from build123d import *

# Parameters (mm, degrees)
ESQUISSE1_W             = 48
ESQUISSE1_H             = 38
BOSS_EXTRU_1_DEPTH      = 8
ESQUISSE4_W             = 14
ESQUISSE4_H             = 15
ENL_V_MAT_EXTRU_2_DEPTH = 8
D_GAGEMENT_M41_D        = 4.3
D_GAGEMENT_M41_DEPTH    = 10
D_GAGEMENT_M41_TIP      = 1.291850331


with BuildPart() as part:
    # Esquisse1 → Boss.-Extru.1 (new body)
    with BuildSketch(Plane.XY):
        Rectangle(ESQUISSE1_W, ESQUISSE1_H)
    extrude(amount=BOSS_EXTRU_1_DEPTH)

    # Esquisse4 → Enlèv. mat.-Extru.2 (cut)
    with BuildSketch(Plane.XY.offset(8)):
        with Locations((17, 0)):
            Rectangle(ESQUISSE4_W, ESQUISSE4_H)
    extrude(amount=-ENL_V_MAT_EXTRU_2_DEPTH, mode=Mode.SUBTRACT)

    # Dégagement M41
    with Locations(Plane(origin=(-20, 14.5, 8), x_dir=(1, 0, 0), z_dir=(0, 0, 1))):
        with Locations((0, 0), (40, 0), (0, -29), (40, -29)):
            Hole(D_GAGEMENT_M41_D / 2, depth=D_GAGEMENT_M41_DEPTH)
            with Locations((0, 0, -(D_GAGEMENT_M41_DEPTH + D_GAGEMENT_M41_TIP / 2))):  # 118° drill point
                Cone(0, D_GAGEMENT_M41_D / 2, D_GAGEMENT_M41_TIP, mode=Mode.SUBTRACT)


solid = part.part
Input: part model. Units: mm. Frame: model coordinates. A direction names the side the tool comes from. Round coordinates to 2 decimals unless told otherwise and drop trailing zeros. Order: outer loops, then holes, each group sorted by start corner. A loop starts at its lowest first (then second) coordinate and runs counter-clockwise, first axis right, second up. Notation, with made-up numbers: (-30.5, 45) - (-6.5, 45) arc R29 ccw to (-6.5, 75) - close; hole circle Ø10 at (61, -31.75). An arc over 180 degrees is marked (long way). Answer as a JSON object with one key per item and string values. Group by question number.
(1) Cut plane B-B (x = -20). Return loops of the section in (y, z), then the cut area to 3 significant figures.
(2) Cut plane C-C (x = 20). Return loops of the section in (y, z).
(3) Cut plane D-D (z = 1.5). Return loops of the section in (x, y).
(4) Cut plane A-A (y = -14.5). Return loops of the section in (x, z).
(5) Draft query along X for faces 3 (the face through (0, 0, 8)), 4 (the face through (-24, 0, 4)), 5 (the face through (24, 13, 4)), 6 (the face through (-19.53, -16.6, 3.94)). Return one class per face: released by +X, released by -X, zero draft, split by the parting line, or undercut.
(6) Reachability of faces 1 (the face through (10, 0, 4)), 2 (the face through (-19.53, 12.4, 3.94)) from +Z, -Z, +X, -X, +Y, -Y: full face, straight path, thin tool, end or side. Return the list, or none.
(7) Material intervals for probe 1 along Y at (x, z) = (20, 4); probe 2 along Y at (x, z) = (-20, 5); probe 3 along Y at (x, z) = (15, 6.5), sorted ascending. Write a range as from..to.
Here are the results:
{
 "1": {"outline": "(-19, 0) - (-16.65, 0) - (-16.65, 8) - (-19, 8) - close; (-12.35, 0) - (12.35, 0) - (12.35, 8) - (-12.35, 8) - close; (16.65, 0) - (19, 0) - (19, 8) - (16.65, 8) - close", "area": "235 mm^2"},
 "2": {"outline": "(-19, 0) - (-16.65, 0) - (-16.65, 8) - (-19, 8) - close; (-12.35, 0) - (-7.5, 0) - (-7.5, 8) - (-12.35, 8) - close; (7.5, 0) - (12.35, 0) - (12.35, 8) - (7.5, 8) - close; (16.65, 0) - (19, 0) - (19, 8) - (16.65, 8) - close"},
 "3": {"outline": "(-24, -19) - (24, -19) - (24, -7.5) - (10, -7.5) - (10, 7.5) - (24, 7.5) - (24, 19) - (-24, 19) - close; hole circle Ø4.3 at (-20, -14.5); hole circle Ø4.3 at (-20, 14.5); hole circle Ø4.3 at (20, -14.5); hole circle Ø4.3 at (20, 14.5)"},
 "4": {"outline": "(-24, 0) - (-22.15, 0) - (-22.15, 8) - (-24, 8) - close; (-17.85, 0) - (17.85, 0) - (17.85, 8) - (-17.85, 8) - close; (22.15, 0) - (24, 0) - (24, 8) - (22.15, 8) - close"},
 "5": {"face 3": "zero draft", "face 4": "released by -X", "face 5": "released by +X", "face 6": "undercut"},
 "6": {"face 1": "+Z, -Z, +X", "face 2": "+Z, -Z"},
 "7": {"probe 1": "y = -19..-16.65, -12.35..-7.5, 7.5..12.35, 16.65..19", "probe 2": "y = -19..-16.65, -12.35..12.35, 16.65..19", "probe 3": "y = -19..-7.5, 7.5..19"}
}
